```python
from build123d import *

# Parameters (mm, degrees)
F0_W     = 60
F0_H     = 60
F2_W     = 60
F2_H     = 60
F5_R     = 5
F6_DEPTH = 5
F7_R     = 7.5
F8_DEPTH = 5
F9_R     = 2


with BuildPart() as f3:
    # F0 (on Front) → F3 section 0
    with BuildSketch(Plane.XZ):
        with Locations((30, -30)):
            Rectangle(F0_W, F0_H)
    # F2 (on offset) → F3 section 1
    with BuildSketch(Plane.XZ.offset(60)):
        with Locations((30, -30)):
            Rectangle(F2_W, F2_H)
    loft()

    # F5 (on offset) → F6 (cut)
    with BuildSketch(Plane.XZ.offset(60)):
        with Locations((30.1493108273, -30.2097292106)):
            Circle(F5_R)
    extrude(amount=-F6_DEPTH, mode=Mode.SUBTRACT)

    # F7 (on Front) → F8 (cut)
    with BuildSketch(Plane.XZ):
        with Locations((47.3982296399, -12.8745916897)):
            Circle(F7_R)
        with Locations((12.4750004448, -12.5)):
            Circle(F7_R)
        with Locations((47.3982296399, -30)):
            Circle(F7_R)
        with Locations((12.2961504385, -30)):
            Circle(F7_R)
        with Locations((47.5, -47.5)):
            Circle(F7_R)
        with Locations((12.2961504385, -47.5)):
            Circle(F7_R)
    extrude(amount=F8_DEPTH, mode=Mode.SUBTRACT)

    # F9
    f9_edges = [f3.edges().sort_by_distance(p)[0] for p in [
        (30, 0, 0),
    ]]
    fillet(f9_edges, radius=F9_R)


solid = f3.part
```
Could you check a few things on this model? Use its own coordinates, in mm. A direction names the side the tool comes from. Round coordinates to 2 decimals unless told otherwise and drop trailing zeros. Order: outer loops, then holes, each group sorted by start corner. A loop starts at its lowest first (then second) coordinate and runs counter-clockwise, first axis right, second up. Notation, with made-up numbers: M -8,19 L 21,19 A14 ccw 21,40 Z; hole C 79.5,39 d1. An arc over 180 degrees is marked long. One line per question, with ' | ' between items. Start each with the question number.
(1) Please list where these lines run through material, in increasing order: line 1 along Z through (x, y) = (47.5, -3.55); line 2 along Y through (x, z) = (15.5, -42); line 3 along Y through (x, z) = (29.5, -29).
(2) Thinking about a two-plate mould opening in X: for faces 1 (the face through (60, -30, -30)), 2 (the face through (22, -60, -23)), 3 (the face through (47, -5, -47)), which applies, +X half, -X half, draft (parallel to the pull), parting line (faces both ways), or undercut?
(3) Suppose I cut it at D-D on x = 9. List the corners of the cut face in (y, z) for me.
(4) Suppose I cut it at C-C on z = -14.5. List the corners of the cut face in (x, y) for me.
(5) Suppose I cut it at B-B on x = 47.5. List the corners of the cut face in (y, z) for me.
(6) Suppose I cut it at A-A on z = -47.5. List the corners of the cut face in (x, y) for me, then the cut area to 3 significant figures.
(7) For P1, Ø12, axis at x = 12.475, z = -12.5, coming from the +Y side, with a flat end and sliding along its axis, tell me the tip position at first contact or that it passes through.
(8) For faces 4 (the face through (26.464, -57.535, -26.83)), 5 (the face through (12, -5, -30)), 6 (the face through (30.42, -0.57, -0.6)), which set-ups out of +Z, -Z, +X, -X, +Y, -Y let a thin tool reach every point of the face, with its end or its side?
Geometry results:
1) line 1: -60 to -55, -40 to -37.5, -22.5 to -20.37, -5.38 to 0 | line 2: -60 to -5 | line 3: -55 to 0
2) face 1: +X half | face 2: draft | face 3: undercut
3) outline: M -60,-60 L 0,-60 L 0,-54.24 L -5,-54.24 L -5,-40.76 L 0,-40.76 L 0,-36.74 L -5,-36.74 L -5,-23.26 L 0,-23.26 L 0,-19.15 L -5,-19.15 L -5,-5.85 L 0,-5.85 L 0,-2 A2 ccw -2,0 L -60,0 Z
4) outline: M 0,-60 L 60,-60 L 60,0 L 54.72,0 L 54.72,-5 L 40.08,-5 L 40.08,0 L 19.7,0 L 19.7,-5 L 5.25,-5 L 5.25,0 L 0,0 Z
5) outline: M -60,-60 L 0,-60 L 0,-55 L -5,-55 L -5,-40 L 0,-40 L 0,-37.5 L -5,-37.5 L -5,-22.5 L 0,-22.5 L 0,-20.37 L -5,-20.37 L -5,-5.38 L 0,-5.38 L 0,-2 A2 ccw -2,0 L -60,0 Z
6) outline: M 0,-60 L 60,-60 L 60,0 L 55,0 L 55,-5 L 40,-5 L 40,0 L 19.8,0 L 19.8,-5 L 4.8,-5 L 4.8,0 L 0,0 Z | area: 3,450 mm²
7) P1: y = -5
8) face 4: -Y | face 5: +Y | face 6: +Z, +X, -X, +Y
